Verification items for the finished model (mm, model axes). A direction names the side the tool comes from. Give positions to 0.01 mm unless a question says otherwise; leave off trailing zeros. Write each loop counter-clockwise with the first axis right and the second up, starting at its lowest first coordinate (ties: lowest second). Pieces come first, ordered by that corner, then holes. Notation, with made-up numbers: (-21, 80) - (-13, 80) arc R22 ccw to (-13, 99) - close; hole circle Ø1 at (-11, 28). An arc over 180 degrees is marked (long way). Answer as a JSON object with one key per item and string values. Group by question number.
Item 1: Sectioned sample at D-D, the plane y = -9.5. Record the boundary of the cut face in (x, z), and give its area (3 significant figures).
Item 2: Sectioned sample at B-B, the plane z = 1.3. Record the boundary of the cut face in (x, y).
Item 3: Draft check along X on faces 1 (the face through (-17.03, -14.15, 1.95)), 2 (the face through (-1.216, -1.115, 1.947)), 3 (the face through (-7.8, -3.7, 3.95)). Enter one of: +X half, -X half, draft (parallel to the pull), parting line (faces both ways), or undercut.
Item 4: Tool access check on faces 4 (the face through (-2.59, -2.34, 1.95)), 5 (the face through (-13.195, -4.73, 1.947)). Record the directions out of +Z, -Z, +X, -X, +Y, -Y that give a thin tool (end or side, any length) a straight path to the whole face; none if there is none.
Item 5: Go/stop test with a flat-tipped pin: pin 1 (1.5 mm diameter, centred on y = -5.5, z = 1, fed in from -X). Record where the tip stops, or that it passes through.
Item 6: Sectioned sample at A-A, the plane y = -0.5. Record the boundary of the cut face in (x, z), and give its area (3 significant figures).
Item 7: Scan lines: line 1 along Y through (x, z) = (0, 1.05); line 2 along X through (y, z) = (-4.5, 2.9); line 3 along X through (y, z) = (-0.5, 3.85). Record each from-to range of solid material in increasing order. Write a range as [from, to].
Item 8: Sectioned sample at C-C, the plane x = -15.5. Record the boundary of the cut face in (y, z), and give its area (3 significant figures).
Solid Edge part; units mm, degrees
sketch "Sketch1" plane through (0, 0, 0) normal (0, 0, 1) x (1, 0, 0)
  line L0 (-2.1713, -2.681) -> (-3.013, -1.9994)
  line L1 (-3.013, -1.9994) -> (-6.8721, -5.1785)
  line L2 (-6.8721, -5.1785) -> (-8.2777, -3.7557)
  line L3 (-15, -13.1578) -> (-19.1075, -15.1675)
  line L4 (0, 3.45) -> (-3.9649, 3.45)
  arc A0 (0, 3.45) -> (-2.1713, -2.681) centre (0, 0) cw
  arc A1 (-15, -13.1578) -> (-8.2777, -3.7557) centre (15.6166, -27.9437) cw
  arc A2 (-19.1076, -15.1675) -> (-3.9649, 3.45) centre (15.6166, -27.9437) cw
  circle A3 centre (0, 0) radius 1.65
extrude "Protrusion1" add sketch "Sketch1" along normal blind 3.95
Geometry check:
{
 "1": {"outline": "(-16.46, 0) - (-12.95, 0) - (-12.95, 3.95) - (-16.46, 3.95) - close", "area": "13.9 mm^2"},
 "2": {"outline": "(-19.11, -15.17) - (-15, -13.16) arc R34 cw to (-8.28, -3.76) - (-6.87, -5.18) - (-3.01, -2) - (-2.17, -2.68) arc R3.45 ccw (long way) to (0, 3.45) - (-3.96, 3.45) arc R37 ccw to start; hole circle Ø3.3 at (0, 0)"},
 "3": {"face 1": "+X half", "face 2": "undercut", "face 3": "draft"},
 "4": {"face 4": "+Z, -Z, -Y", "face 5": "+Z, -Z, -X, +Y"},
 "5": {"pin 1": "x = -14.36"},
 "6": {"outline": "(-9.2, 0) - (-1.57, 0) - (-1.57, 3.95) - (-9.2, 3.95) - close; (1.57, 0) - (3.41, 0) - (3.41, 3.95) - (1.57, 3.95) - close", "area": "37.4 mm^2"},
 "7": {"line 1": "[-3.45, -1.65], [1.65, 3.45]", "line 2": "[-13.01, -9.01], [-7.54, -6.05]", "line 3": "[-9.2, -1.57], [1.57, 3.41]"},
 "8": {"outline": "(-13.4, 0) - (-7.92, 0) - (-7.92, 3.95) - (-13.4, 3.95) - close", "area": "21.6 mm^2"}
}
